Verification items for this drawing (mm, ordinates from the low corner). A direction names the side the tool comes from. Round coordinates to 2 decimals unless told otherwise and drop trailing zeros. Loops run counter-clockwise (first coordinate to the right, second up) from the corner with the lowest first, then second, coordinate; pieces in that order, holes last. Notation, with made-up numbers: M 89.25,-35.5 L 143.25,-35.5 A13 ccw 143.25,-24.5 Z; hole C -3.5,82 d2. An arc over 180 degrees is marked long. Use one line per item in the form item = value. Start each with the question number.
1. Material ranges on line 1 (Y direction, x = 2.85, z = 5); line 2 (Z direction, x = 3.35, y = 1); line 3 (Z direction, x = 0.45, y = 2), recorded low to high.
2. Cross-section at A-A (x = 3). Record the boundary of the cut face in (y, z), then the cut area to 3 significant figures.
3. Cross-section at B-B (z = 22). Record the boundary of the cut face in (x, y), then the cut area to 3 significant figures.
4. Go/stop test with flat-tipped pins: pin 1 (2 mm diameter, centred on x = 3.5, z = 9.5, fed in from -Y); pin 2 (1.5 mm diameter, centred on y = 1.5, z = 28, fed in from +X); pin 3 (2 mm diameter, centred on x = 4.5, y = 5, fed in from +Z); pin 4 (3 mm diameter, centred on x = 1, z = 7, fed in from -Y). Record where each tip stops, or that it passes through.
5. Set-up check for the marked faces 1 and 2: record each of +Z, -Z, +X, -X, +Y, -Y from which the full face is reachable in a straight line by a thin tool's end or side.
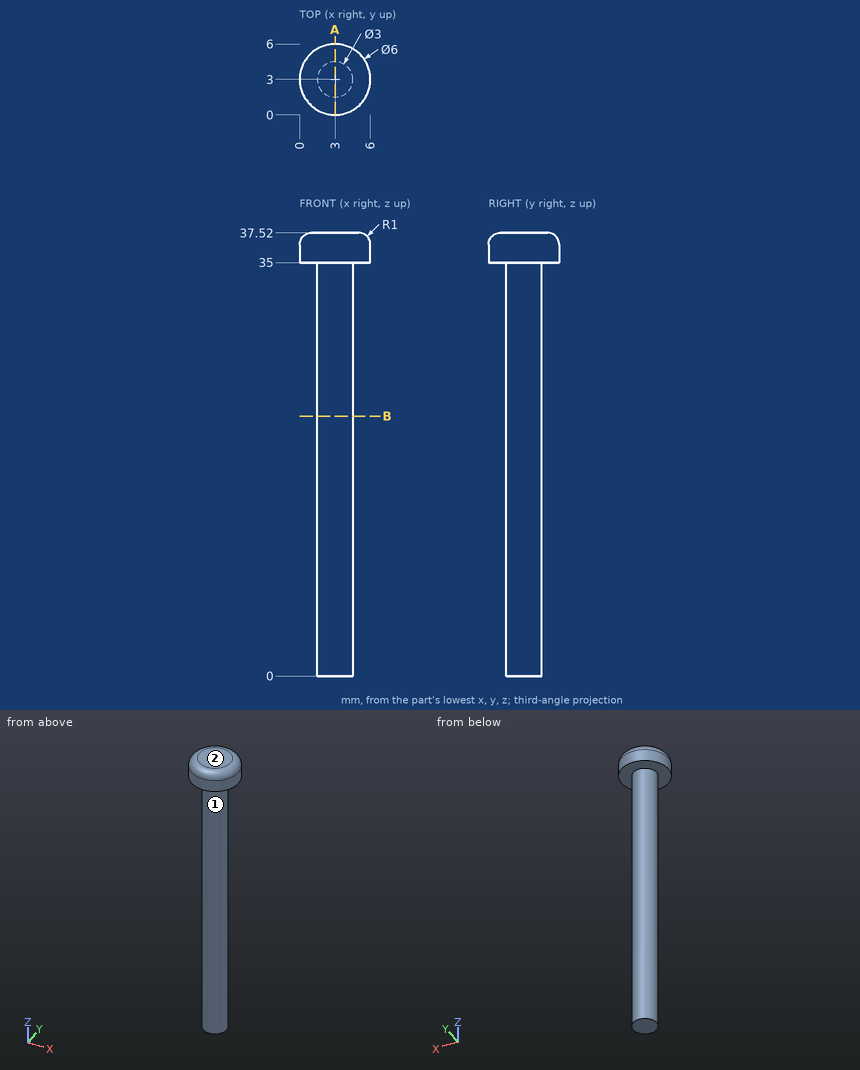
Reported:
q1.line_1 = 1.51 to 4.49
q1.line_2 = 35 to 37.52
q1.line_3 = 35 to 37.19
q2.outline = M 0,35 L 1.5,35 L 1.5,0 L 4.5,0 L 4.5,35 L 6,35 L 6,36.52 A1 ccw 5,37.52 L 1,37.52 A1 ccw 0,36.52 Z
q2.area = 120 mm²
q3.outline = C 3,3 d3
q3.area = 7.07 mm²
q4.pin_1 = 1.5
q4.pin_2 = 4.3
q4.pin_3 = 37.52
q4.pin_4 = 1.59
q5.face_1 = -Z
q5.face_2 = +Z, +X, -X, +Y, -Y
